Autodesk Inventor part; units mm, degrees
ref_plane "Arbeitsebene2" through (2.25, 10, 0) normal (0, 1, 0) x (1, 0, 0)
ref_plane "YZ Plane" through (0, 0, 0) normal (1, 0, 0) x (0, 1, 0)
ref_plane "XZ Plane" through (0, 0, 0) normal (0, 1, 0) x (-1, 0, 0)
sketch "Skizze1" plane through (0, 0, 0) normal (0, 0, 1) x (1, 0, 0)
  line L0 (0, 0) -> (11.5, 0)
  line L1 (11.5, 0) -> (11.5, 20)
  line L2 (11.5, 20) -> (0, 20)
  line L3 (0, 20) -> (0, 0)
  line L4 (2.25, 20) -> (9.25, 20)
  line L5 (9.25, 20) -> (9.25, 21.4)
  line L6 (9.25, 21.4) -> (2.25, 21.4)
  line L7 (2.25, 21.4) -> (2.25, 20)
  line L8 (2.2583, 0) -> (10.4927, 0)
  line L9 (9.25, 0) -> (2.25, 0)
  line L10 (2.25, 0) -> (2.25, -1.4)
  line L11 (2.25, -1.4) -> (9.25, -1.4)
  line L12 (9.25, -1.4) -> (9.25, 0)
  dimension "d0" = 11.5
  dimension "d1" = 20
  dimension "d4" = 7
  dimension "d5" = 1.4
  dimension "d6" = 2.25
  dimension "d7" = 2.25
extrude "Extrusion1" add sketch "Skizze1" along normal blind 13.3
ref_plane "Arbeitsebene2" through (2.25, 10, 0) normal (0, 1, 0) x (1, 0, 0)
sketch "Skizze2" plane through (0, 0, 13.3) normal (0, 0, 1) x (1, 0, 0)
  line L0 (9.25, 21.4) -> (2.25, 21.4)
  line L1 (0, 20) -> (0, 0)
  line L2 (2.25, -1.4) -> (9.25, -1.4)
  line L3 (11.5, 0) -> (11.5, 20)
  line L4 (2.9, 18.15) -> (8.6, 18.15)
  line L5 (9.6, 17.15) -> (9.6, 2.85)
  line L6 (8.6, 1.85) -> (2.9, 1.85)
  line L7 (1.9, 2.85) -> (1.9, 17.15)
  line L8 (2.9, 18.15) -> (1.9, 17.15)
  line L9 (8.6, 18.15) -> (9.6, 17.15)
  line L10 (9.6, 2.85) -> (8.6, 1.85)
  line L11 (2.9, 1.85) -> (1.9, 2.85)
  point P0 (1.9, 18.15)
  point P1 (9.6, 1.85)
  point P2 (9.6, 18.15)
  point P3 (1.9, 1.85)
  dimension "d8" = 1.9
  dimension "d9" = 1.9
  dimension "d10" = 3.25
  dimension "d11" = 3.25
  dimension "d12" = 1
  dimension "d13" = 1
  dimension "d14" = 1
  dimension "d15" = 1
  dimension "d16" = 1
  dimension "d17" = 1
  dimension "d18" = 1
  dimension "d19" = 1
extrude "Extrusion2" cut sketch "Skizze2" against normal blind 0.7
sketch "Skizze4" plane through (0, 0, 0) normal (0, 0, -1) x (-1, 0, 0)
  line L0 (-2.25, 21.4) -> (-2.25, 20)
  line L1 (-9.25, 21.4) -> (-2.25, 21.4)
  line L2 (-9.25, 20) -> (-9.25, 21.4)
  line L3 (-9.25, -1.4) -> (-9.25, 0)
  line L4 (-2.25, -1.4) -> (-9.25, -1.4)
  line L5 (-2.25, 0) -> (-2.25, -1.4)
  line L6 (-9.25, 20.6) -> (-2.25, 20.6)
  dimension "d32" = 0.8
extrude "Extrusion3" add sketch "Skizze4" along normal blind 4.5
sketch "Skizze5" plane through (2.25, 21.4, 13.3) normal (0, 1, 0) x (1, 0, 0)
  line L0 (7, 17.8) -> (7, 0)
  line L1 (0, 17.8) -> (7, 17.8)
  line L2 (0, 17.8) -> (7, 17.8)
  line L3 (7, 17.8) -> (7, 16.5)
  line L4 (7, 16.5) -> (0, 16.5)
  line L5 (0, 16.5) -> (0, 17.8)
  point P0 (-2.25, 13.3)
  dimension "d36" = 1.3
extrude "Extrusion4" add sketch "Skizze5" along normal blind 1
chamfer "Fase1" distance 1 angle 45 1 edges at (5.75, 22.4, -4.5)
mirror "Spiegeln1" about plane through (2.25, 10, 0) normal (0, 1, 0) of "Extrusion4", "Fase1", "Extrusion3"
properties part number "motor_shaft"
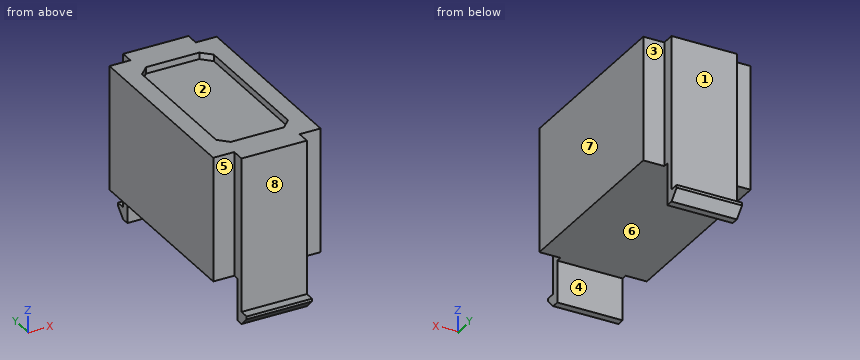
Read the model definition and answer for the solid it produces. Units are mm, in the model's axes. Face numbers are marked on the shaded views. A direction names the side the tool comes from. Coordinates: 2 decimals unless noted, no trailing zeros. Write each loop counter-clockwise with the first axis right and the second up, starting at its lowest first coordinate (ties: lowest second). Pieces come first, ordered by that corner, then holes. Notation, with made-up numbers: (39, 65.5) -> (72, 65.5) arc R12 ccw to (72, 70.5) -> close; hole circle Ø3 at (-17.5, 9.5). An arc over 180 degrees is marked (long way). Write item = value, one per line.
(1) Section D-D on y = 10.25 is taken. Write down the section's boundary in (x, z).
From the geometry:
outline = (0, 0) -> (11.5, 0) -> (11.5, 13.3) -> (9.6, 13.3) -> (9.6, 12.6) -> (1.9, 12.6) -> (1.9, 13.3) -> (0, 13.3) -> close
(2) Given pin 1 Ø1.9 at (y, z) = (21.5, 6.5) entering from -X; pin 2 Ø0.7 at (y, z) = (-1.5, 0.5) entering from +X; pin 3 Ø0.7 at (x, z) = (11, 8) entering from -Y, each flat-ended and moving along its own axis, determine where each tip first touches the part or whether it passes through.
From the geometry:
pin_1 = 2.25
pin_2 = 9.25
pin_3 = 0
(3) Section C-C on y = 2.5 is taken. Write down the section's boundary in (x, z).
From the geometry:
outline = (0, 0) -> (11.5, 0) -> (11.5, 13.3) -> (9.25, 13.3) -> (9.25, 12.6) -> (2.25, 12.6) -> (2.25, 13.3) -> (0, 13.3) -> close
(4) Which of the six approach directions +Z, -Z, +X, -X, +Y, -Y give full straight-line access (tool end or side, diameter ignored) to the marked faces 1, 2, 3, 4 and 5?
From the geometry:
face_1 = +Z, +X, -X, +Y
face_2 = +Z
face_3 = +Z, -Z, +X, +Y
face_4 = -Z, +X, -X
face_5 = +Z, -Z, -X, -Y
(5) Section A-A on z = 9 is taken. Write down the section's boundary in (x, y), plus the area to 3 significant figures.
From the geometry:
outline = (0, 0) -> (2.25, 0) -> (2.25, -1.4) -> (9.25, -1.4) -> (9.25, 0) -> (11.5, 0) -> (11.5, 20) -> (9.25, 20) -> (9.25, 21.4) -> (2.25, 21.4) -> (2.25, 20) -> (0, 20) -> close
area = 250 mm2
(6) Straight lines are drawn through the part: L1, parallel to Y at x = 7.25, z = -1.5; L2, parallel to Y at x = 9, z = 5.5; L3, parallel to Z at x = 4.25, y = 16.25. For each, find the intervals that lie inside material, in ascending order. Write a range as from..to.
From the geometry:
L1 = -1.4..-0.6, 20.6..21.4
L2 = -1.4..21.4
L3 = 0..12.6
(7) Section B-B on x = 5.75 is taken. Write down the section's boundary in (y, z), plus the area to 3 significant figures.
From the geometry:
outline = (-2.4, -3.5) -> (-1.4, -4.5) -> (-0.6, -4.5) -> (-0.6, 0) -> (20.6, 0) -> (20.6, -4.5) -> (21.4, -4.5) -> (22.4, -3.5) -> (22.4, -3.2) -> (21.4, -3.2) -> (21.4, 13.3) -> (18.15, 13.3) -> (18.15, 12.6) -> (1.85, 12.6) -> (1.85, 13.3) -> (-1.4, 13.3) -> (-1.4, -3.2) -> (-2.4, -3.2) -> close
area = 301 mm2
(8) For a pull along Y with two mould halves and no side action, classify the marked faces 6, 7 and 8 as +Y half, -Y half, draft (parallel to the pull), parting line (faces both ways), or undercut.
From the geometry:
face_6 = undercut
face_7 = draft
face_8 = -Y half
